```python
from build123d import *

# Parameters (mm, degrees)
SKETCH1_W           = 500
SKETCH1_H           = 500
BOSS_EXTRUDE1_DEPTH = 5
SKETCH2_R           = 125
CUT_EXTRUDE1_DEPTH  = 1


with BuildPart() as part:
    # Sketch1 → Boss-Extrude1 (new, symmetric)
    with BuildSketch(Plane(origin=(0, 0, 0), x_dir=(1, 0, 0), z_dir=(0, 1, 0))):
        Rectangle(SKETCH1_W, SKETCH1_H)
    extrude(amount=BOSS_EXTRUDE1_DEPTH, both=True)

    # Sketch2 → Cut-Extrude1 (cut)
    with BuildSketch(Plane(origin=(0, 5, 0), x_dir=(1, 0, 0), z_dir=(0, 1, 0))):
        with Locations(Location((0, 0, 0), (0, 0, 270))):
            Circle(SKETCH2_R)
    extrude(amount=-CUT_EXTRUDE1_DEPTH, mode=Mode.SUBTRACT)


solid = part.part
```
The model under review builds one solid part; all positions refer to its coordinate system, in mm. A direction names the side the tool comes from. Round coordinates to 2 decimals unless told otherwise and drop trailing zeros. Order: outer loops, then holes, each group sorted by start corner. A loop starts at its lowest first (then second) coordinate and runs counter-clockwise, first axis right, second up. Notation, with made-up numbers: (-31, 20) -> (3, 20) arc R17 ccw to (3, 36) -> close; hole circle Ø4 at (-4, 85.25). An arc over 180 degrees is marked (long way). Use a Markdown table: item, result.
Q1. Clearance check with a flat-ended pin moving along its axis: P1, Ø4, axis at x = -31.5, z = 11.5, coming from the +Y side. State where the tip first meets the part, or that it passes through.
Values:
| item | result |
|---|---|
| P1 | stops at y = 4 |
Q2. We need section B-B on x = 0. Write out the cut boundary in (y, z).
Values:
| item | result |
|---|---|
| outline | (-5, -250) -> (5, -250) -> (5, -125) -> (4, -125) -> (4, 125) -> (5, 125) -> (5, 250) -> (-5, 250) -> close |
Q3. Tool access review of faces 3 (the flat face through (2, 4, -2)), 4 (the flat face through (-3, -5, -4)): name each direction out of +Z, -Z, +X, -X, +Y, -Y from which nothing blocks a thin tool from reaching the whole face with its end or side.
Values:
| item | result |
|---|---|
| face 3 | +Y |
| face 4 | +Z, -Z, +X, -X, -Y |
Q4. For line 1 (X direction, y = 4.6, z = 0); line 2 (Y direction, x = 74.5, z = 46), list the stretches that pass through material, from the lowest coordinate up.
Values:
| item | result |
|---|---|
| line 1 | x = -250 to -125, 125 to 250 |
| line 2 | y = -5 to 4 |
Q5. Mouldability with a two-part tool opening along X and no side actions: class faces 1 (the cylindrical face through (5.5, 4.51, -124.88)), 2 (the flat face through (-59, 5, -115)) as +X half, -X half, draft (parallel to the pull), parting line (faces both ways), or undercut.
Values:
| item | result |
|---|---|
| face 1 | undercut |
| face 2 | draft |
Q6. We need section A-A on z = 0. Write out the cut boundary in (x, y), then the cut area to 3 significant figures.
Values:
| item | result |
|---|---|
| outline | (-250, -5) -> (250, -5) -> (250, 5) -> (125, 5) -> (125, 4) -> (-125, 4) -> (-125, 5) -> (-250, 5) -> close |
| area | 4,750 mm^2 |
